Autodesk Inventor part; units mm, degrees
ref_plane "YZ Plane" through (0, 0, 0) normal (1, 0, 0) x (0, 1, 0)
ref_plane "XZ Plane" through (0, 0, 0) normal (0, 1, 0) x (-1, 0, 0)
ref_plane "XY Plane" through (0, 0, 0) normal (0, 0, 1) x (1, 0, 0)
sketch "Sketch1" plane through (0, 0, 0) normal (0, 1, 0) x (-1, 0, 0)
  circle A0 centre (0, 0) radius 3.5
  circle A1 centre (0, 0) radius 2.1
  dimension "d0" = 7
  dimension "d1" = 4.2
extrude "Extrusion1" add sketch "Sketch1" along normal blind 8.9
sketch "Sketch2" plane through (0, 8.9, 0) normal (0, 1, 0) x (1, 0, 0)
  circle A0 centre (0, 0) radius 3.5
  circle A1 centre (0, 0) radius 3
  dimension "d4" = 6
extrude "Extrusion2" cut sketch "Sketch2" against normal blind 0.25
sketch "Sketch3" plane through (0, 0, 0) normal (0, -1, 0) x (1, 0, 0)
  circle A0 centre (0, 0) radius 3.5
  circle A1 centre (0, 0) radius 3
extrude "Extrusion3" cut sketch "Sketch3" against normal blind 0.25
properties part number "InnerBearingSpacer"
Model file for the job. Use its own axes, mm. A direction names the side the tool comes from. Round coordinates to 2 decimals unless told otherwise and drop trailing zeros. Write each loop counter-clockwise with the first axis right and the second up, starting at its lowest first coordinate (ties: lowest second). Pieces come first, ordered by that corner, then holes. Notation, with made-up numbers: (56, 33.5) -> (74, 33.5) arc R21 cw to (74, 51.5) -> close; hole circle Ø4 at (79.25, 77.25). An arc over 180 degrees is marked (long way). Answer as CSV lines item,"result".
1. Slice it at A-A, the plane x = 0. List the corners of the cut face in (y, z).
Resolved:
outline,"(0, -3) -> (0.25, -3) -> (0.25, -3.5) -> (8.65, -3.5) -> (8.65, -3) -> (8.9, -3) -> (8.9, -2.1) -> (0, -2.1) -> close; (0, 2.1) -> (8.9, 2.1) -> (8.9, 3) -> (8.65, 3) -> (8.65, 3.5) -> (0.25, 3.5) -> (0.25, 3) -> (0, 3) -> close"
2. Tool access for faces 1 (the face through (3, 0.25, 1)), 2 (the face through (-1.3, 8.9, -2)), 3 (the face through (3, 8.65, -1)): list every direction of +Z, -Z, +X, -X, +Y, -Y with a clear straight run to the whole face (end or side of a thin tool).
Resolved:
face 1,"-Y"
face 2,"+Z, -Z, +X, -X, +Y"
face 3,"+Y"
3. Slice it at D-D, the plane y = 3.25. List the corners of the cut face in (x, z), plus the area to 3 significant figures.
Resolved:
outline,"circle Ø7 at (0, 0); hole circle Ø4.2 at (0, 0)"
area,"24.6 mm²"
4. Slice it at C-C, the plane z = 2.75. List the corners of the cut face in (x, y), plus the area to 3 significant figures.
Resolved:
outline,"(-2.17, 0.25) -> (-1.2, 0.25) -> (-1.2, 0) -> (1.2, 0) -> (1.2, 0.25) -> (2.17, 0.25) -> (2.17, 8.65) -> (1.2, 8.65) -> (1.2, 8.9) -> (-1.2, 8.9) -> (-1.2, 8.65) -> (-2.17, 8.65) -> close"
area,"37.6 mm²"
5. Mould opens along Z. For faces 4 (the face through (-1.3, 0, -2)), 5 (the face through (-2.003, 4.388, -0.631)), 6 (the face through (-3.233, 4.391, 1.341)) say: +Z half, -Z half, draft (parallel to the pull), parting line (faces both ways), or undercut.
Resolved:
face 4,"draft"
face 5,"undercut"
face 6,"parting line"
6. Drill centre lines: line 1 (Z direction, x = 0, y = 2.5); line 2 (Z direction, x = 0.75, y = 4.75). Where is each one in solid material? Low to high.
Resolved:
line 1,"-3.5 to -2.1, 2.1 to 3.5"
line 2,"-3.42 to -1.96, 1.96 to 3.42"
7. Slice it at B-B, the plane z = 0. List the corners of the cut face in (x, y).
Resolved:
outline,"(-3.5, 0.25) -> (-3, 0.25) -> (-3, 0) -> (-2.1, 0) -> (-2.1, 8.9) -> (-3, 8.9) -> (-3, 8.65) -> (-3.5, 8.65) -> close; (2.1, 0) -> (3, 0) -> (3, 0.25) -> (3.5, 0.25) -> (3.5, 8.65) -> (3, 8.65) -> (3, 8.9) -> (2.1, 8.9) -> close"
8. Pin check, flat tips, straight feed: pin 1 Ø2 at (x, y) = (2, 2) entering from +Z; pin 2 Ø1 at (x, y) = (-2, 5) entering from -Z; pin 3 Ø1.5 at (x, y) = (-2.5, 3) entering from -Z. Stop position of each tip, or through.
Resolved:
pin 1,"z = 3.35"
pin 2,"z = -3.16"
pin 3,"z = -3.03"
